```python
from build123d import *

# Parameters (mm, degrees)
SKETCH1_R               = 20
BOSS_EXTRUDE1_DEPTH     = 4
SKETCH2_R               = 7.5
BOSS_EXTRUDE2_DEPTH     = 14
SKETCH3_R               = 3.5
CUT_EXTRUDE1_DEPTH      = 14
SKETCH5_R               = 1.5
CUT_EXTRUDE2_DEPTH      = 21
CUT_EXTRUDE2_DEPTH_BACK = 21
FILLET1_R               = 2
SKETCH6_R               = 2.1
CUT_EXTRUDE3_DEPTH      = 5


with BuildPart() as part:
    # Sketch1 → Boss-Extrude1 (new body)
    with BuildSketch(Plane(origin=(0, 0, 0), x_dir=(1, 0, 0), z_dir=(0, 1, 0))):
        Circle(SKETCH1_R)
    extrude(amount=BOSS_EXTRUDE1_DEPTH)

    # Sketch2 → Boss-Extrude2 (add)
    with BuildSketch(Plane(origin=(0, 4, 0), x_dir=(1, 0, 0), z_dir=(0, 1, 0))):
        Circle(SKETCH2_R)
    extrude(amount=BOSS_EXTRUDE2_DEPTH)

    # Sketch3 → Cut-Extrude1 (cut)
    with BuildSketch(Plane(origin=(0, 18, 0), x_dir=(1, 0, 0), z_dir=(0, 1, 0))):
        Circle(SKETCH3_R)
    extrude(amount=-CUT_EXTRUDE1_DEPTH, mode=Mode.SUBTRACT)

    # Sketch5 → Cut-Extrude2 (cut, two sides)
    with BuildSketch(Plane.XY) as cut_extrude2_sk:
        with Locations((0, 13)):
            Circle(SKETCH5_R)
    extrude(amount=CUT_EXTRUDE2_DEPTH, mode=Mode.SUBTRACT)
    extrude(cut_extrude2_sk.sketch, amount=-CUT_EXTRUDE2_DEPTH_BACK, mode=Mode.SUBTRACT)

    # Fillet1
    fillet1_edges = [part.edges().sort_by_distance(p)[0] for p in [
        (-7.5, 4, 0),
    ]]
    fillet(fillet1_edges, radius=FILLET1_R)

    # Sketch6 → Cut-Extrude3 (cut, through all)
    with BuildSketch(Plane(origin=(0, 4, 0), x_dir=(1, 0, 0), z_dir=(0, 1, 0))):
        with Locations((10.606601718, 10.606601718)):
            Circle(SKETCH6_R)
        with Locations((-10.606601718, 10.606601718)):
            Circle(SKETCH6_R)
        with Locations((-10.606601718, -10.606601718)):
            Circle(SKETCH6_R)
        with Locations((10.606601718, -10.606601718)):
            Circle(SKETCH6_R)
    extrude(amount=-CUT_EXTRUDE3_DEPTH, mode=Mode.SUBTRACT)


solid = part.part
```
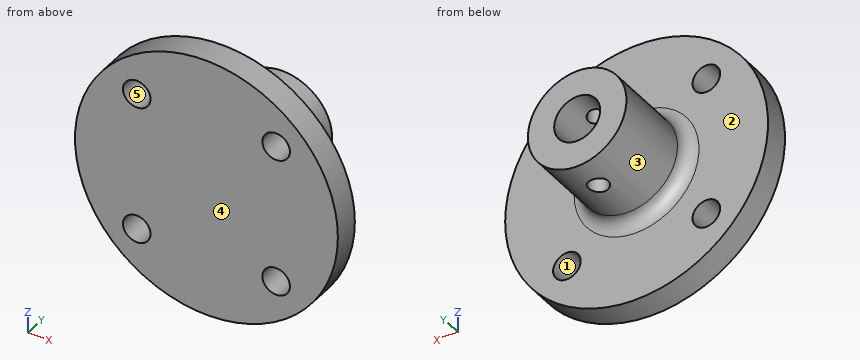
Can you work these out from the model? Positions are in its coordinate system, mm. Face numbers are marked on the shaded views. A direction names the side the tool comes from. Round coordinates to 2 decimals unless told otherwise and drop trailing zeros. Loops run counter-clockwise (first coordinate to the right, second up) from the corner with the lowest first, then second, coordinate; pieces in that order, holes last.
Item 1: Suppose I cut it at B-B, the plane y = 13. Write out the boundary of the cut face in (x, z), then the cut area to 3 significant figures.
Item 2: If we mould it in two halves opening along X, with no side actions, what happens to the marked faces 3, 4 and 5? For each: +X half, -X half, draft (parallel to the pull), parting line (faces both ways), or undercut.
Item 3: Suppose I cut it at C-C, the plane z = -11.5. Write out the boundary of the cut face in (x, y).
Item 4: Suppose I cut it at A-A, the plane x = 0. Write out the boundary of the cut face in (y, z), then the cut area to 3 significant figures.
Item 5: Which directions (+Z, -Z, +X, -X, +Y, -Y) give clear straight access to the entire face, cutting with the end or side of a thin tool? Please do the marked faces 1 and 2.
Item 6: Please list where these lines run through material, in increasing order: L1, parallel to X at y = 15, z = 0; L2, parallel to Z at x = 11.5, y = 3.25.
Item 7: Suppose I cut it at D-D, the plane z = 0. Write out the boundary of the cut face in (x, y), then the cut area to 3 significant figures.
Item 8: Will these pins go through, and if not, where does the flat tip stop? pin 1 Ø2.5 at (x, z) = (10.61, 10.61) entering from -Y; pin 2 Ø10 at (y, z) = (4.5, 8.5) entering from +X; pin 3 Ø3 at (x, z) = (14, 7) entering from +Y; pin 4 Ø10 at (y, z) = (10.5, -4) entering from +X.
Reported:
1. outline: (-1.5, -7.35) - (-1.5, -3.16) arc R3.5 cw to (-1.5, 3.16) - (-1.5, 7.35) arc R7.5 ccw to start; (1.5, -7.35) arc R7.5 ccw to (1.5, 7.35) - (1.5, 3.16) arc R3.5 cw to (1.5, -3.16) - close
1. area: 114 mm2
2. face 3: parting line
2. face 4: draft
2. face 5: undercut
3. outline: (-16.36, 0) - (-12.51, 0) - (-12.51, 4) - (-16.36, 4) - close; (-8.71, 0) - (8.71, 0) - (8.71, 4) - (-8.71, 4) - close; (12.51, 0) - (16.36, 0) - (16.36, 4) - (12.51, 4) - close
4. outline: (0, -20) - (4, -20) - (4, -9.5) arc R2 cw to (6, -7.5) - (11.5, -7.5) - (11.5, -3.5) - (4, -3.5) - (4, 3.5) - (11.5, 3.5) - (11.5, 7.5) - (6, 7.5) arc R2 cw to (4, 9.5) - (4, 20) - (0, 20) - close; (14.5, -7.5) - (18, -7.5) - (18, -3.5) - (14.5, -3.5) - close; (14.5, 3.5) - (18, 3.5) - (18, 7.5) - (14.5, 7.5) - close
4. area: 250 mm2
5. face 1: +Y, -Y
5. face 2: +Y
6. L1: x = -7.5 to -3.5, 3.5 to 7.5
6. L2: z = -16.36 to -12.51, -8.71 to 8.71, 12.51 to 16.36
7. outline: (-20, 0) - (20, 0) - (20, 4) - (9.5, 4) arc R2 cw to (7.5, 6) - (7.5, 18) - (3.5, 18) - (3.5, 4) - (-3.5, 4) - (-3.5, 18) - (-7.5, 18) - (-7.5, 6) arc R2 cw to (-9.5, 4) - (-20, 4) - close
7. area: 274 mm2
8. pin 1: passes through
8. pin 2: stops at x = 19.69
8. pin 3: stops at y = 4
8. pin 4: stops at x = 7.5
